Geometry: final body of the model. Coordinates: model frame, mm. A direction names the side the tool comes from. Give positions to 0.01 mm unless a question says otherwise; leave off trailing zeros. Order: outer loops, then holes, each group sorted by start corner. A loop starts at its lowest first (then second) coordinate and runs counter-clockwise, first axis right, second up. Notation, with made-up numbers: (16.25, 70) -> (45.25, 70) arc R26 ccw to (45.25, 85) -> close; hole circle Ø6 at (77.25, 54.5). An arc over 180 degrees is marked (long way). Write item = value, one per line.
```python
from build123d import *

# Parameters (mm, degrees)
BOSS_EXTRUDE1_DEPTH        = 41.5
SKETCH2_W                  = 3.459033884
SKETCH2_H                  = 7.669300129
BOSS_EXTRUDE2_DEPTH        = 4.5
FILLET1_R                  = 1.2
FILLET2_R                  = 0.7
SKETCH3_W                  = 1.676518228
SKETCH3_H                  = 0.644745983
CUT_EXTRUDE1_DEPTH         = 0.2
FILLET3_R                  = 0.15
LPATTERN1_COUNT            = 3
LPATTERN1_PITCH            = 1
FILLET3_OF_LPATTERN1_R     = 0.15
LPATTERN1_COL_COUNT        = 3
LPATTERN1_COL_PITCH        = 1
FILLET3_OF_LPATTERN1_COL_R = 0.15


with BuildPart() as part:
    # Sketch1 → Boss-Extrude1 (new body)
    with BuildSketch(Plane(origin=(0, 0, 0), x_dir=(1, 0, 0), z_dir=(0, 1, 0))):
        Polygon((0.878746859, -0.34499804), (5.591575223, -0.34499804), (5.591575223, 1.95500196), (7.288815202, 1.95500196), (8.091575223, 3.966300559), (-1.621253141, 3.966300559), (-0.81849312, 1.95500196), (0.878746859, 1.95500196), align=None)
    extrude(amount=BOSS_EXTRUDE1_DEPTH)

    # Sketch2 → Boss-Extrude2 (add)
    with BuildSketch(Plane.XY.offset(0.34499804)):
        with Locations((3.235161041, 37.399269449)):
            Rectangle(SKETCH2_W, SKETCH2_H)
    extrude(amount=BOSS_EXTRUDE2_DEPTH)

    # Fillet1
    fillet1_edges = [part.edges().sort_by_distance(p)[0] for p in [
        (1.505644099, 41.233919514, 2.59499804),
        (1.505644099, 33.564619385, 2.59499804),
        (4.964677983, 33.564619385, 2.59499804),
        (4.964677983, 41.233919514, 2.59499804),
    ]]
    fillet(fillet1_edges, radius=FILLET1_R)

    # Fillet2
    fillet2_edges = [part.edges().sort_by_distance(p)[0] for p in [
        (3.235161041, 41.233919514, 4.84499804),
        (4.964677983, 37.399269449, 4.84499804),
        (1.505644099, 37.399269449, 4.84499804),
        (3.235161041, 33.564619385, 4.84499804),
        (4.613206121, 33.916091248, 4.84499804),
        (1.857115961, 33.916091248, 4.84499804),
        (1.857115961, 40.882447651, 4.84499804),
        (4.613206121, 40.882447651, 4.84499804),
    ]]
    fillet(fillet2_edges, radius=FILLET2_R)

    # Sketch3 → Cut-Extrude1 (cut)
    with BuildSketch(Plane.XY.offset(4.84499804)):
        with Locations((3.235161041, 37.399269449)):
            Rectangle(SKETCH3_W, SKETCH3_H)
    cut_extrude1 = extrude(amount=-CUT_EXTRUDE1_DEPTH, mode=Mode.SUBTRACT)

    # Fillet3
    fillet3_edges = [part.edges().sort_by_distance(p)[0] for p in [
        (2.396901927, 37.076896458, 4.74499804),
        (2.396901927, 37.721642441, 4.74499804),
        (4.073420155, 37.721642441, 4.74499804),
        (4.073420155, 37.076896458, 4.74499804),
    ]]
    fillet(fillet3_edges, radius=FILLET3_R)

    # LPattern1: Cut-Extrude1 ×3
    with Locations(*[(0, i * LPATTERN1_PITCH, 0) for i in range(1, LPATTERN1_COUNT)]):
        add(cut_extrude1, mode=Mode.SUBTRACT)

    # Fillet3 of LPattern1
    fillet3_of_lpattern1_edges = [part.edges().sort_by_distance(p)[0] for p in [
        (2.396901927, 38.076896458, 4.74499804),
        (2.396901927, 38.721642441, 4.74499804),
        (4.073420155, 38.721642441, 4.74499804),
        (4.073420155, 38.076896458, 4.74499804),
        (2.396901927, 39.076896458, 4.74499804),
        (2.396901927, 39.721642441, 4.74499804),
        (4.073420155, 39.721642441, 4.74499804),
        (4.073420155, 39.076896458, 4.74499804),
    ]]
    fillet(fillet3_of_lpattern1_edges, radius=FILLET3_OF_LPATTERN1_R)

    # LPattern1 col: Cut-Extrude1 ×3
    with Locations(*[(0, -i * LPATTERN1_COL_PITCH, 0) for i in range(1, LPATTERN1_COL_COUNT)]):
        add(cut_extrude1, mode=Mode.SUBTRACT)

    # Fillet3 of LPattern1 col
    fillet3_of_lpattern1_col_edges = [part.edges().sort_by_distance(p)[0] for p in [
        (2.396901927, 36.076896458, 4.74499804),
        (2.396901927, 36.721642441, 4.74499804),
        (4.073420155, 36.721642441, 4.74499804),
        (4.073420155, 36.076896458, 4.74499804),
        (2.396901927, 35.076896458, 4.74499804),
        (2.396901927, 35.721642441, 4.74499804),
        (4.073420155, 35.721642441, 4.74499804),
        (4.073420155, 35.076896458, 4.74499804),
    ]]
    fillet(fillet3_of_lpattern1_col_edges, radius=FILLET3_OF_LPATTERN1_COL_R)


solid = part.part
```
1) Line query: line 1 (Z direction, x = 0.5, y = 34) (3 decimals); line 2 (Z direction, x = 2, y = 6) (3 decimals); line 3 (X direction, y = 10.5, z = 0.25). Output: solid intervals per line, ascending. Write a range as from..to.
Check sheet entries:
line_1 = -3.966..-1.955
line_2 = -3.966..0.345
line_3 = 0.88..5.59
2) Section query C-C (x = 6.25). Output: boundary loops of the cut face in (y, z) (3 decimals).
Check sheet entries:
outline = (0, -3.966) -> (41.5, -3.966) -> (41.5, -1.955) -> (0, -1.955) -> close
3) Reachability of faces 1 (the face through (3, 41.234, 2)), 2 (the face through (4.965, 37, 2)), 3 (the face through (1.506, 37, 2)) from +Z, -Z, +X, -X, +Y, -Y: full face, straight path, thin tool, end or side. Return the list, or none.
Check sheet entries:
face_1 = +Z, +X, -X, +Y
face_2 = +Z, +X, +Y, -Y
face_3 = +Z, -X, +Y, -Y
4) Section query A-A (y = 17). Output: boundary loops of the cut face in (x, z) (1 decimal), plus the area to 3 significant figures.
Check sheet entries:
outline = (-1.6, -4) -> (8.1, -4) -> (7.3, -2) -> (5.6, -2) -> (5.6, 0.3) -> (0.9, 0.3) -> (0.9, -2) -> (-0.8, -2) -> close
area = 28.8 mm²
5) First-contact query: P1, Ø0.5, axis at x = 0.5, y = 13, coming from the +Z side (3 decimals); P2, Ø3, axis at x = 5.5, z = -2, coming from the -Y side; P3, Ø5, axis at y = 30.5, z = 2, coming from the +X side; P4, Ø1, axis at x = 7, z = 3, coming from the -Y side. Flat tips, straight axial feed; report the tip coordinate or a pass-through.
Check sheet entries:
P1 = -1.955
P2 = 0
P3 = 5.59
P4 = through
6) Section query D-D (z = -0.75). Output: boundary loops of the cut face in (x, y), plus the area to 3 significant figures.
Check sheet entries:
outline = (0.88, 0) -> (5.59, 0) -> (5.59, 41.5) -> (0.88, 41.5) -> close
area = 196 mm²
7) Section query B-B (z = 3.5). Output: boundary loops of the cut face in (x, y), plus the area to 3 significant figures.
Check sheet entries:
outline = (1.51, 34.76) arc R1.2 ccw to (2.71, 33.56) -> (3.76, 33.56) arc R1.2 ccw to (4.96, 34.76) -> (4.96, 40.03) arc R1.2 ccw to (3.76, 41.23) -> (2.71, 41.23) arc R1.2 ccw to (1.51, 40.03) -> close
area = 25.3 mm²
